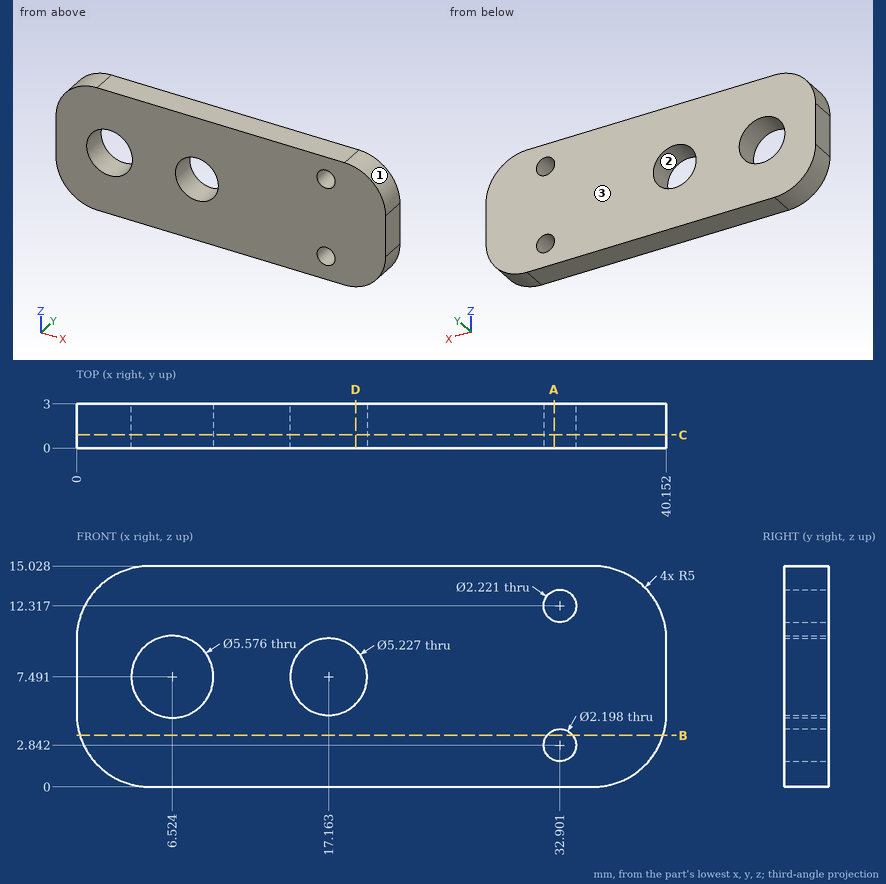
Can you work these out from the drawing? Everything is in mm from the part's minimum corner. Round coordinates to 2 decimals unless told otherwise and drop trailing zeros. Order: outer loops, then holes, each group sorted by start corner. A loop starts at its lowest first (then second) coordinate and runs counter-clockwise, first axis right, second up. Notation, with made-up numbers: (-19.5, 86.25) - (-10.5, 86.25) arc R20 cw to (-10.5, 125.25) - close; hole circle Ø4 at (47, 75.25). An arc over 180 degrees is marked (long way). Answer in a Markdown table with one row per item.
(1) Suppose I cut it at C-C, the plane y = 0.9. Please give me the cut outline in (x, z) (1 decimal).
From the geometry:
| item | result |
|---|---|
| outline | (0, 5) arc R5 ccw to (5, 0) - (35.2, 0) arc R5 ccw to (40.2, 5) - (40.2, 10) arc R5 ccw to (35.2, 15) - (5, 15) arc R5 ccw to (0, 10) - close; hole circle Ø5.6 at (6.5, 7.5); hole circle Ø5.2 at (17.2, 7.5); hole circle Ø2.2 at (32.9, 2.8); hole circle Ø2.2 at (32.9, 12.3) |
(2) Suppose I cut it at A-A, the plane x = 32.5. Please give me the cut outline in (y, z) (1 decimal).
From the geometry:
| item | result |
|---|---|
| outline | (0, 0) - (3, 0) - (3, 1.8) - (0, 1.8) - close; (0, 3.9) - (3, 3.9) - (3, 11.3) - (0, 11.3) - close; (0, 13.4) - (3, 13.4) - (3, 15) - (0, 15) - close |
(3) For P1, Ø1, axis at y = 0.5, z = 12.5, coming from the -X side (1 decimal); P2, Ø7, axis at x = 6.52, z = 7.49, coming from the -Y side, each with a flat end and sliding along its axis, tell me the tip position at first contact or that it passes through.
From the geometry:
| item | result |
|---|---|
| P1 | stops at x = 0.4 |
| P2 | stops at y = 0 |
(4) Please list where these lines run through material, in increasing order: L1, parallel to Z at x = 33, y = 2.65; L2, parallel to X at y = 0.2, z = 9; L3, parallel to X at y = 2.15, z = 7.25 (1 decimal). Write a range as from..to.
From the geometry:
| item | result |
|---|---|
| L1 | z = 0..1.75, 3.94..11.21, 13.42..15.03 |
| L2 | x = 0..4.18, 8.87..15.03, 19.3..40.15 |
| L3 | x = 0..3.7, 9.3..14.6, 19.8..40.2 |
(5) If we mould it in two halves opening along Z, with no side actions, what happens to the marked faces 1, 2 and 3? For each: released by +Z, released by -Z, zero draft, split by the parting line, or undercut.
From the geometry:
| item | result |
|---|---|
| face 1 | released by +Z |
| face 2 | undercut |
| face 3 | zero draft |
(6) Suppose I cut it at D-D, the plane x = 19. Please give me the cut outline in (y, z).
From the geometry:
| item | result |
|---|---|
| outline | (0, 0) - (3, 0) - (3, 5.63) - (0, 5.63) - close; (0, 9.35) - (3, 9.35) - (3, 15.03) - (0, 15.03) - close |
(7) Suppose I cut it at B-B, the plane z = 3.5. Please give me the cut outline in (x, y), plus the area to 3 significant figures.
From the geometry:
| item | result |
|---|---|
| outline | (0.23, 0) - (32.02, 0) - (32.02, 3) - (0.23, 3) - close; (33.78, 0) - (39.92, 0) - (39.92, 3) - (33.78, 3) - close |
| area | 114 mm2 |
